Input: part model. Units: mm. Frame: model coordinates. A direction names the side the tool comes from. Round coordinates to 2 decimals unless told otherwise and drop trailing zeros. Write each loop counter-clockwise with the first axis right and the second up, starting at its lowest first coordinate (ties: lowest second). Pieces come first, ordered by that corner, then holes. Notation, with made-up numbers: (39, 32) -> (65, 32) arc R19 cw to (65, 48) -> close; hole circle Ø10 at (-9, -5). An arc over 180 degrees is marked (long way). Write item = value, one per line.
```python
from build123d import *

# Parameters (mm, degrees)
F0_W     = 150
F0_H     = 140
F0_W_2   = 18.4
F0_H_2   = 35.8
F0_W_3   = 13
F0_H_3   = 14.5
F0_W_4   = 40
F0_H_4   = 10
F0_W_5   = 22.4
F0_W_6   = 125
F0_H_5   = 80
F0_W_7   = 12.4
F0_H_6   = 12.4
F1_DEPTH = 2.5
F2_DEPTH = 3.5
F3_W     = 150
F3_H     = 140
F3_W_2   = 18.4
F3_H_2   = 35.8
F3_W_3   = 13
F3_H_3   = 14.5
F3_W_4   = 40
F3_H_4   = 10
F3_W_5   = 125
F3_H_5   = 80
F4_DEPTH = 3
F5_W     = 150
F5_H     = 140
F5_W_2   = 10.5
F5_H_2   = 6.7
F6_DEPTH = 6.5


with BuildPart() as f1:
    # F0 (on Top) → F1 (new body)
    with BuildSketch(Plane.XY):
        with Locations((-4.5338094234, 6.6955923945)):
            Rectangle(F0_W, F0_H)
        with Locations((-60.8338094234, -41.4044076055)):
            Rectangle(F0_W_2, F0_H_2, mode=Mode.SUBTRACT)
        with Locations((-34.5338094234, -43.4044076055)):
            Rectangle(F0_W_3, F0_H_3, mode=Mode.SUBTRACT)
        with Locations((-4.6338094234, -26.8044076055)):
            Rectangle(F0_W_4, F0_H_4, mode=Mode.SUBTRACT)
        with Locations((-4.5338094234, -43.4044076055)):
            Rectangle(F0_W_3, F0_H_3, mode=Mode.SUBTRACT)
        with Locations((25.4661905766, -43.4044076055)):
            Rectangle(F0_W_3, F0_H_3, mode=Mode.SUBTRACT)
        with Locations((51.7661905766, -41.4044076055)):
            Rectangle(F0_W_5, F0_H_2, mode=Mode.SUBTRACT)
        with Locations((-4.5338094234, 23.1955923945)):
            Rectangle(F0_W_6, F0_H_5, mode=Mode.SUBTRACT)
        with Locations((-60.8338094234, -41.4044076055)):
            Rectangle(F0_W_2, F0_H_2)
        with Locations((-60.8338094234, -50.1044076055)):
            Rectangle(F0_W_7, F0_H_6, mode=Mode.SUBTRACT)
        with Locations((-60.8338094234, -32.7044076055)):
            Rectangle(F0_W_7, F0_H_6, mode=Mode.SUBTRACT)
        with Locations((51.7661905766, -41.4044076055)):
            Rectangle(F0_W_5, F0_H_2)
        with Locations((51.7661905766, -50.1044076055)):
            Rectangle(F0_W_7, F0_H_6, mode=Mode.SUBTRACT)
        with Locations((51.7661905766, -32.7044076055)):
            Rectangle(F0_W_7, F0_H_6, mode=Mode.SUBTRACT)
        with Locations((-4.6338094234, -26.8044076055)):
            Rectangle(F0_W_4, F0_H_4)
    extrude(amount=F1_DEPTH)

    # F0 (on Top) → F2 (join)
    with BuildSketch(Plane.XY):
        with Locations((-4.5338094234, 6.6955923945)):
            Rectangle(F0_W, F0_H)
        with Locations((-60.8338094234, -41.4044076055)):
            Rectangle(F0_W_2, F0_H_2, mode=Mode.SUBTRACT)
        with Locations((-34.5338094234, -43.4044076055)):
            Rectangle(F0_W_3, F0_H_3, mode=Mode.SUBTRACT)
        with Locations((-4.6338094234, -26.8044076055)):
            Rectangle(F0_W_4, F0_H_4, mode=Mode.SUBTRACT)
        with Locations((-4.5338094234, -43.4044076055)):
            Rectangle(F0_W_3, F0_H_3, mode=Mode.SUBTRACT)
        with Locations((25.4661905766, -43.4044076055)):
            Rectangle(F0_W_3, F0_H_3, mode=Mode.SUBTRACT)
        with Locations((51.7661905766, -41.4044076055)):
            Rectangle(F0_W_5, F0_H_2, mode=Mode.SUBTRACT)
        with Locations((-4.5338094234, 23.1955923945)):
            Rectangle(F0_W_6, F0_H_5, mode=Mode.SUBTRACT)
        with Locations((-60.8338094234, -41.4044076055)):
            Rectangle(F0_W_2, F0_H_2)
        with Locations((-60.8338094234, -50.1044076055)):
            Rectangle(F0_W_7, F0_H_6, mode=Mode.SUBTRACT)
        with Locations((-60.8338094234, -32.7044076055)):
            Rectangle(F0_W_7, F0_H_6, mode=Mode.SUBTRACT)
        with Locations((51.7661905766, -41.4044076055)):
            Rectangle(F0_W_5, F0_H_2)
        with Locations((51.7661905766, -50.1044076055)):
            Rectangle(F0_W_7, F0_H_6, mode=Mode.SUBTRACT)
        with Locations((51.7661905766, -32.7044076055)):
            Rectangle(F0_W_7, F0_H_6, mode=Mode.SUBTRACT)
    extrude(amount=F2_DEPTH)

    # F3 (on face) → F4 (join)
    with BuildSketch(Plane.XY.offset(3.5)):
        with Locations((-4.5338094234, 6.6955923945)):
            Rectangle(F3_W, F3_H)
        with Locations((-60.8338094234, -41.4044076055)):
            Rectangle(F3_W_2, F3_H_2, mode=Mode.SUBTRACT)
        with Locations((-34.5338094234, -43.4044076055)):
            Rectangle(F3_W_3, F3_H_3, mode=Mode.SUBTRACT)
        with Locations((-4.6338094234, -26.8044076055)):
            Rectangle(F3_W_4, F3_H_4, mode=Mode.SUBTRACT)
        with Locations((-4.5338094234, -43.4044076055)):
            Rectangle(F3_W_3, F3_H_3, mode=Mode.SUBTRACT)
        with Locations((25.4661905766, -43.4044076055)):
            Rectangle(F3_W_3, F3_H_3, mode=Mode.SUBTRACT)
        with Locations((51.7661905766, -41.4044076055)):
            Rectangle(F3_W_2, F3_H_2, mode=Mode.SUBTRACT)
        with Locations((-4.5338094234, 23.1955923945)):
            Rectangle(F3_W_5, F3_H_5, mode=Mode.SUBTRACT)
    extrude(amount=F4_DEPTH)

    # F5 (on face) → F6 (join)
    with BuildSketch(Plane.XY.offset(6.5)):
        with Locations((-4.5338094234, 6.6955923945)):
            Rectangle(F5_W, F5_H)
        Polygon((-67.0338094234, -23.5044076055), (-67.0338094234, -16.8044076055), (-67.0338094234, 63.1955923945), (-8.0338094234, 63.1955923945), (-8.0338094234, 73.1955923945), (14.9661905766, 73.1955923945), (14.9661905766, 63.1955923945), (57.9661905766, 63.1955923945), (57.9661905766, -16.8044076055), (57.9661905766, -23.5044076055), (60.9661905766, -23.5044076055), (60.9661905766, -59.3044076055), (42.5661905766, -59.3044076055), (-51.6338094234, -59.3044076055), (-70.0338094234, -59.3044076055), (-70.0338094234, -23.5044076055), align=None, mode=Mode.SUBTRACT)
        with Locations((-61.7838094234, -20.1544076055)):
            Rectangle(F5_W_2, F5_H_2)
        with Locations((52.7161905766, -20.1544076055)):
            Rectangle(F5_W_2, F5_H_2)
    extrude(amount=F6_DEPTH)


solid = f1.part
```
1) Cut plane C-C (z = 10). Return the cut outline in (x, y).
Solutions:
outline = (-79.53, -63.3) -> (70.47, -63.3) -> (70.47, 76.7) -> (-79.53, 76.7) -> close; hole (-70.03, -59.3) -> (60.97, -59.3) -> (60.97, -23.5) -> (47.47, -23.5) -> (47.47, -16.8) -> (57.97, -16.8) -> (57.97, 63.2) -> (14.97, 63.2) -> (14.97, 73.2) -> (-8.03, 73.2) -> (-8.03, 63.2) -> (-67.03, 63.2) -> (-67.03, -16.8) -> (-56.53, -16.8) -> (-56.53, -23.5) -> (-70.03, -23.5) -> close
2) Line query: L1, parallel to X at y = -45.5, z = 1.5; L2, parallel to Y at x = -9.5, z = 5.5; L3, parallel to Y at x = -36.5, z = 5.5. Output: solid intervals per line, ascending. Write a range as from..to.
Solutions:
L1 = -79.53..-67.03, -54.63..-41.03, -28.03..-11.03, 1.97..18.97, 31.97..45.57, 57.97..70.47
L2 = -63.3..-50.65, -36.15..-31.8, -21.8..-16.8, 63.2..76.7
L3 = -63.3..-50.65, -36.15..-16.8, 63.2..76.7
3) Access query for faces 1 (the face through (52, -26.504, 2)), 2 (the face through (-4, -59.304, 9)). Directions: +Z, -Z, +X, -X, +Y, -Y. A direction counts if a zero-diameter tool reaches every point of the face in a straight line with its end or side. Return the directions, or none.
Solutions:
face_1 = +Z, -Z
face_2 = +Z
4) Cut plane D-D (x = -15). Return the cut outline in (y, z).
Solutions:
outline = (-63.3, 0) -> (-16.8, 0) -> (-16.8, 6.5) -> (-21.8, 6.5) -> (-21.8, 2.5) -> (-31.8, 2.5) -> (-31.8, 6.5) -> (-59.3, 6.5) -> (-59.3, 13) -> (-63.3, 13) -> close; (63.2, 0) -> (76.7, 0) -> (76.7, 13) -> (63.2, 13) -> close
5) Cut plane B-B (y = 50). Return the cut outline in (x, z), and give its area (3 significant figures).
Solutions:
outline = (-79.53, 0) -> (-67.03, 0) -> (-67.03, 13) -> (-79.53, 13) -> close; (57.97, 0) -> (70.47, 0) -> (70.47, 13) -> (57.97, 13) -> close
area = 325 mm^2
6) Draft query along Y for faces 3 (the face through (-6, 76.696, 6)), 4 (the face through (1.966, -44, 3)), 5 (the face through (-22, 64, 13)). Return one class per face: +Y half, -Y half, draft (parallel to the pull), parting line (faces both ways), or undercut.
Solutions:
face_3 = +Y half
face_4 = undercut
face_5 = draft
7) Cut plane A-A (x = 5). Return the cut outline in (y, z).
Solutions:
outline = (-63.3, 0) -> (-16.8, 0) -> (-16.8, 6.5) -> (-21.8, 6.5) -> (-21.8, 2.5) -> (-31.8, 2.5) -> (-31.8, 6.5) -> (-59.3, 6.5) -> (-59.3, 13) -> (-63.3, 13) -> close; (63.2, 0) -> (76.7, 0) -> (76.7, 13) -> (73.2, 13) -> (73.2, 6.5) -> (63.2, 6.5) -> close
8) First-contact query: P1, Ø5, axis at x = -2, y = 68, coming from the +Z side. Flat tip, straight axial feed; report the tip coordinate or a pass-through.
Solutions:
P1 = 6.5
